from build123d import *

# Parameters (mm, degrees)
SKETCH001_W     = 43.9111261831
SKETCH001_H     = 56
EXTRUDE_DEPTH   = 10.9
POCKET001_DEPTH = 43.9121261831
SKETCH003_W     = 31.1652
SKETCH003_H     = 8.6
POCKET002_DEPTH = 10.901
SKETCH006_R     = 2.5
POCKET004_DEPTH = 10.9


with BuildPart() as part:
    # Sketch001 (on Face7 of Pocket) → Extrude (new body)
    with BuildSketch(Plane(origin=(66.9555630915, 66.3037746961, 29.39946064), x_dir=(-1, 0, 0), z_dir=(0, 0, 1))):
        with Locations((17, 28)):
            Rectangle(SKETCH001_W, SKETCH001_H)
    extrude(amount=EXTRUDE_DEPTH)

    # Sketch002 (on Face4 of Extrude) → Pocket001 (cut, through all)
    with BuildSketch(Plane.YZ.offset(71.9111261831)):
        with BuildLine():
            Line((10.3037746961, 29.39946064), (34.0037746961, 29.39946064))
            ThreePointArc((34.0037746961, 29.39946064), (33.1543764894, 31.4500781776), (31.1037524304, 32.29946064))
            Line((22.0537746961, 32.29946064), (31.1037524304, 32.29946064))
            ThreePointArc((17.4537746961, 36.8994600326), (18.8010836591, 33.6467691735), (22.0537746961, 32.29946064))
            Line((17.4537746961, 36.8994600326), (17.4537746961, 40.29946064))
            Line((10.3037746961, 40.29946064), (17.4537746961, 40.29946064))
            Line((10.3037746961, 40.29946064), (10.3037746961, 29.39946064))
        make_face()
    extrude(amount=-POCKET001_DEPTH, mode=Mode.SUBTRACT)

    # Sketch003 (on Face7 of Pocket001) → Pocket002 (cut, through all)
    with BuildSketch(Plane.XY.offset(40.29946064)):
        with Locations((49.9555387865, 21.7537746961)):
            Rectangle(SKETCH003_W, SKETCH003_H)
    extrude(amount=-POCKET002_DEPTH, mode=Mode.SUBTRACT)

    # Sketch006 (on Face7 of Pocket002) → Pocket004 (cut)
    with BuildSketch(Plane.XY.offset(40.29946064)):
        with Locations((49.9555630915, 38.4537746961)):
            Circle(SKETCH006_R)
    extrude(amount=-POCKET004_DEPTH, mode=Mode.SUBTRACT)


solid = part.part
Geometry check sheet. Reference: the model listing, model coordinates, mm. A direction names the side the tool comes from. Give positions to 0.01 mm unless a question says otherwise; leave off trailing zeros. Order: outer loops, then holes, each group sorted by start corner. A loop starts at its lowest first (then second) coordinate and runs counter-clockwise, first axis right, second up.
1) Cross-section at A-A (z = 33.75). Record the boundary of the cut face in (x, y), then the cut area to 3 significant figures.
Results are:
outline: (28, 18.7) - (34.37, 18.7) - (34.37, 26.05) - (65.54, 26.05) - (65.54, 18.7) - (71.91, 18.7) - (71.91, 66.3) - (28, 66.3) - close; hole circle Ø5 at (49.96, 38.45)
area: 1,840 mm2
2) Cross-section at C-C (y = 40). Record the boundary of the cut face in (x, z), then the cut area to 3 significant figures.
Results are:
outline: (28, 29.4) - (47.99, 29.4) - (47.99, 40.3) - (28, 40.3) - close; (51.92, 29.4) - (71.91, 29.4) - (71.91, 40.3) - (51.92, 40.3) - close
area: 436 mm2
3) Cross-section at D-D (x = 33). Record the boundary of the cut face in (y, z), then the cut area to 3 significant figures.
Results are:
outline: (17.45, 36.9) arc R4.6 ccw to (22.05, 32.3) - (31.1, 32.3) arc R2.9 cw to (34, 29.4) - (66.3, 29.4) - (66.3, 40.3) - (17.45, 40.3) - close
area: 482 mm2
4) Gauge pin test, flat ends, axial feed: pin 1 (8 mm diameter, centred on x = 49.96, y = 38.45, fed in from +Z); pin 2 (2.5 mm diameter, centred on x = 55.5, z = 36, fed in from -Y); pin 3 (7 mm diameter, centred on x = 49.5, y = 28, fed in from -Z). Record the tip position at first contact, or that the pin passes through.
Results are:
pin 1: stops at z = 40.3
pin 2: stops at y = 26.05
pin 3: stops at z = 32.27
5) Cross-section at B-B (x = 50). Record the boundary of the cut face in (y, z), then the cut area to 3 significant figures.
Results are:
outline: (26.05, 32.3) - (31.1, 32.3) arc R2.9 cw to (34, 29.4) - (35.95, 29.4) - (35.95, 40.3) - (26.05, 40.3) - close; (40.95, 29.4) - (66.3, 29.4) - (66.3, 40.3) - (40.95, 40.3) - close
area: 363 mm2
6) Material ranges on probe 1 along X at (y, z) = (25, 35.5); probe 2 along Z at (x, y) = (70.5, 25); probe 3 along Y at (x, z) = (44, 33.75), recorded low to high.
Results are:
probe 1: x = 28 to 34.37, 65.54 to 71.91
probe 2: z = 32.3 to 40.3
probe 3: y = 26.05 to 66.3
7) Draft check along X on faces 1 (the flat face through (50, 66.304, 35)), 2 (the flat face through (34.373, 22, 36)), 3 (the flat face through (28, 42, 35)). Enter one of: released by +X, released by -X, zero draft, split by the parting line, or undercut.
Results are:
face 1: zero draft
face 2: undercut
face 3: released by -X
8) Tool access check on faces 4 (the flat face through (50, 28, 32.299)), 5 (the flat face through (71.911, 42, 35)), 6 (the flat face through (50, 26.054, 36)). Record the directions out of +Z, -Z, +X, -X, +Y, -Y that give a thin tool (end or side, any length) a straight path to the whole face; none if there is none.
Results are:
face 4: -Z, +X, -X, -Y
face 5: +Z, -Z, +X, +Y, -Y
face 6: +Z, -Z, -Y
